Can you work these out from the model? Positions are in its coordinate system, mm. A direction names the side the tool comes from. Give positions to 0.01 mm unless a question says otherwise; leave off trailing zeros. Write each loop counter-clockwise with the first axis right and the second up, starting at its lowest first coordinate (ties: lowest second). Pieces come first, ordered by that corner, then holes.
1. I'm going to push flat-ended pins straight in: pin 1 (4 mm diameter, centred on y = 124, z = -25, fed in from -X); pin 2 (1 mm diameter, centred on y = 203.5, z = -11.5, fed in from +X); pin 3 (5 mm diameter, centred on y = 193, z = 10, fed in from +X). Where does each tip first touch, or does it pass through?
2. On a 3-axis mill with a long thin cutter (end or side, diameter ignored), from which of +Z, -Z, +X, -X, +Y, -Y can I reach the whole of each face in a straight line? I mean faces 4 (the cylindrical face through (-15.62, 3.94, 3.47)), 5 (the flat face through (-26.66, 120.404, 15.106)), 6 (the flat face through (-10, 118, -37.641)). Say none if no direction works.
3. Suppose I cut it at D-D (x = 26.5). Please give me the cut outline in (y, z).
4. Suppose I cut it at B-B (x = 0). Please give me the cut outline in (y, z), and give its area (3 significant figures).
5. Suppose I cut it at C-C (z = 21). Please give me the cut outline in (x, y), and give its area (3 significant figures).
6. Thinking about a two-plate mould opening in Y: for faces 1 (the flat face through (-29.86, 118.32, -17.56)), 2 (the flat face through (0, 120, 30.641)), 3 (the flat face through (-1, 240, -2)), which applies, pulls with the +Y half, pulls with the -Y half, needs draft (parallel to the pull), parting line crosses it, or undercut?
7. Suppose I cut it at A-A (y = 180). Please give me the cut outline in (x, z).
8. If I drill on probe 1 along X at (y, z) = (2, 0); probe 2 along Y at (x, z) = (13.5, -28); probe 3 along Z at (x, y) = (10, 214), over which ranges is the centre line in solid material (lowest first)?
```python
from build123d import *

# Parameters (mm, degrees)
BOSS_EXTRUDE1_DEPTH = 240
SHELL1_START        = 8
SHELL1_DEPTH        = 228
CUT_EXTRUDE1_REACH  = 248.205
SKETCH2_R           = 16


# Read off the part's stored shape, not the designer's step: Shell1
with BuildPart() as part:
    # Sketch1 → Boss-Extrude1 (new body)
    with BuildSketch(Plane(origin=(0, 0, 0), x_dir=(1, 0, 0), z_dir=(0, 1, 0))):
        Polygon((40, 0), (20, 34.641016151), (-20, 34.641016151), (-40, 0), (-20, -34.641016151), (20, -34.641016151), align=None)
        Polygon((-12, 34.641016151), (-8, 34.641016151), (-4, 37.641016151), (-16, 37.641016151), align=None)
        Polygon((4, 37.641016151), (16, 37.641016151), (12, 34.641016151), (8, 34.641016151), align=None)
    extrude(amount=BOSS_EXTRUDE1_DEPTH)

    # Shell1 outline → Shell1 (cut)
    with BuildSketch(Plane(origin=(0, 0, 0), x_dir=(1, 0, 0), z_dir=(0, 1, 0)).offset(SHELL1_START)):
        Polygon((-17.690598923, -30.641016151), (17.690598923, -30.641016151), (35.381197846, 0), (17.690598923, 30.641016151), (-17.690598923, 30.641016151), (-35.381197846, 0), align=None)
    extrude(amount=SHELL1_DEPTH, mode=Mode.SUBTRACT)

    # Sketch2 → Cut-Extrude1 (cut, up to next)
    with BuildSketch(Plane.XZ, mode=Mode.PRIVATE) as cut_extrude1_sk1:
        with Locations(Location((0, 0, 0), (0, 0, 270))):
            Circle(SKETCH2_R)
    cut_extrude1_tool1 = extrude(cut_extrude1_sk1.sketch, amount=-CUT_EXTRUDE1_REACH, mode=Mode.PRIVATE) & part.part
    add(cut_extrude1_tool1.solids().sort_by_distance((0, 0, 0))[0], mode=Mode.SUBTRACT)


solid = part.part
```
Checks:
1. pin 1: stops at x = -26.72
1. pin 2: stops at x = 33.65
1. pin 3: stops at x = 35.67
2. face 4: -Y
2. face 5: none
2. face 6: -Z, +X, -X, +Y, -Y
3. outline: (0, -23.38) - (240, -23.38) - (240, 23.38) - (0, 23.38) - close; hole (8, -15.38) - (236, -15.38) - (236, 15.38) - (8, 15.38) - close
4. outline: (0, -34.64) - (240, -34.64) - (240, 34.64) - (0, 34.64) - (0, 16) - (8, 16) - (8, 30.64) - (236, 30.64) - (236, -30.64) - (8, -30.64) - (8, -16) - (0, -16) - close
4. area: 2,400 mm2
5. outline: (-27.88, 0) - (27.88, 0) - (27.88, 240) - (-27.88, 240) - close; hole (-23.26, 8) - (23.26, 8) - (23.26, 236) - (-23.26, 236) - close
5. area: 2,780 mm2
6. face 1: needs draft
6. face 2: undercut
6. face 3: pulls with the +Y half
7. outline: (-40, 0) - (-20, -34.64) - (-12, -34.64) - (-16, -37.64) - (-4, -37.64) - (-8, -34.64) - (8, -34.64) - (4, -37.64) - (16, -37.64) - (12, -34.64) - (20, -34.64) - (40, 0) - (20, 34.64) - (-20, 34.64) - close; hole (-35.38, 0) - (-17.69, -30.64) - (17.69, -30.64) - (35.38, 0) - (17.69, 30.64) - (-17.69, 30.64) - close
8. probe 1: x = -40 to -16, 16 to 40
8. probe 2: y = 0 to 8, 236 to 240
8. probe 3: z = -37.64 to -30.64, 30.64 to 34.64
